Here's how the part is built. I have some questions about the finished solid (model axes, mm). Face numbers are marked on the shaded views. A direction names the side the tool comes from. Round coordinates to 2 decimals unless told otherwise and drop trailing zeros. Write each loop counter-clockwise with the first axis right and the second up, starting at its lowest first coordinate (ties: lowest second). Pieces come first, ordered by that corner, then holes. Notation, with made-up numbers: (68, 53.25) -> (82, 53.25) arc R4 ccw to (82, 57.25) -> close; hole circle Ø3 at (73.5, 71). An arc over 180 degrees is marked (long way). Answer as CSV lines item,"result".
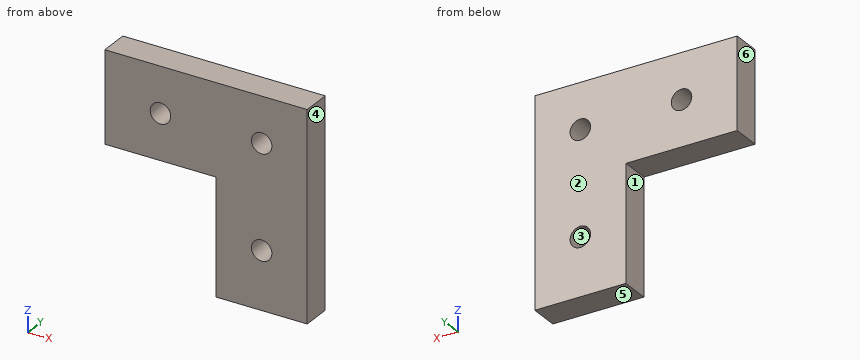
```python
from build123d import *

# Parameters (mm, degrees)
SKETCH1_W           = 20
SKETCH1_H           = 25.4
SKETCH1_W_2         = 44.45
SKETCH1_H_2         = 20
BOSS_EXTRUDE1_DEPTH = 6.35
SKETCH2_R           = 2.25
CUT_EXTRUDE1_DEPTH  = 6.35


with BuildPart() as part:
    # Sketch1 → Boss-Extrude1 (new body)
    with BuildSketch(Plane(origin=(0, 0, 0), x_dir=(1, 0, 0), z_dir=(0, 1, 0))):
        with Locations((34.45, 32.7)):
            Rectangle(SKETCH1_W, SKETCH1_H)
        with Locations((22.225, 10)):
            Rectangle(SKETCH1_W_2, SKETCH1_H_2)
    extrude(amount=BOSS_EXTRUDE1_DEPTH)

    # Sketch2 → Cut-Extrude1 (cut)
    with BuildSketch(Plane(origin=(0, 6.35, 0), x_dir=(1, 0, 0), z_dir=(0, 1, 0))):
        with Locations(Location((12.225, 10, 0), (0, 0, 270))):
            Circle(SKETCH2_R)
        with Locations(Location((34.45, 10, 0), (0, 0, 270))):
            Circle(SKETCH2_R)
        with Locations(Location((34.45, 32.7, 0), (0, 0, 270))):
            Circle(SKETCH2_R)
    extrude(amount=-CUT_EXTRUDE1_DEPTH, mode=Mode.SUBTRACT)


solid = part.part
```
1. If we mould it in two halves opening along X, with no side actions, what happens to the marked faces 3, 4, 5 and 6? For each: released by +X, released by -X, zero draft, split by the parting line, or undercut.
Numbers:
face 3,"undercut"
face 4,"released by +X"
face 5,"zero draft"
face 6,"released by -X"
2. On a 3-axis mill with a long thin cutter (end or side, diameter ignored), from which of +Z, -Z, +X, -X, +Y, -Y can I reach the whole of each face in a straight line? I mean the marked faces 1 and 2. Say none if no direction works.
Numbers:
face 1,"-Z, -X, +Y, -Y"
face 2,"+Z, -Z, +X, -X, +Y"
3. Suppose I cut it at C-C on z = -10. Please give me the cut outline in (x, y) (3 decimals).
Numbers:
outline,"(0, 0) -> (9.975, 0) -> (9.975, 6.35) -> (0, 6.35) -> close; (14.475, 0) -> (32.2, 0) -> (32.2, 6.35) -> (14.475, 6.35) -> close; (36.7, 0) -> (44.45, 0) -> (44.45, 6.35) -> (36.7, 6.35) -> close"
4. Suppose I cut it at B-B on x = 34.45. Please give me the cut outline in (y, z), and give its area (3 significant figures).
Numbers:
outline,"(0, -45.4) -> (6.35, -45.4) -> (6.35, -34.95) -> (0, -34.95) -> close; (0, -30.45) -> (6.35, -30.45) -> (6.35, -12.25) -> (0, -12.25) -> close; (0, -7.75) -> (6.35, -7.75) -> (6.35, 0) -> (0, 0) -> close"
area,"231 mm^2"
5. If I drill on line 1 (X direction, y = 3.75, z = -10) (3 decimals); line 2 (Z direction, x = 34.5, y = 1); line 3 (Z direction, x = 33.5, y = 5), over which ranges is the centre line in solid material (lowest first)?
Numbers:
line 1,"x = 0 to 9.975, 14.475 to 32.2, 36.7 to 44.45"
line 2,"z = -45.4 to -34.95, -30.45 to -12.25, -7.75 to 0"
line 3,"z = -45.4 to -34.74, -30.66 to -12.04, -7.96 to 0"
6. Suppose I cut it at A-A on z = -32.7. Please give me the cut outline in (x, y).
Numbers:
outline,"(24.45, 0) -> (32.2, 0) -> (32.2, 6.35) -> (24.45, 6.35) -> close; (36.7, 0) -> (44.45, 0) -> (44.45, 6.35) -> (36.7, 6.35) -> close"
7. Suppose I cut it at D-D on y = 1.5. Please give me the cut outline in (x, z) (3 decimals), and give its area (3 significant figures).
Numbers:
outline,"(0, -20) -> (24.45, -20) -> (24.45, -45.4) -> (44.45, -45.4) -> (44.45, 0) -> (0, 0) -> close; hole circle Ø4.5 at (12.225, -10); hole circle Ø4.5 at (34.45, -32.7); hole circle Ø4.5 at (34.45, -10)"
area,"1,350 mm^2"
8. For pin 1 Ø3 at (y, z) = (3, -28.5) entering from -X, with a flat end and sliding along its axis, tell me the tip position at first contact or that it passes through.
Numbers:
pin 1,"stops at x = 24.45"
